from build123d import *

# Parameters (mm, degrees)
SKETCH1_W           = 94.925
SKETCH1_H           = 94.024999972
BOSS_EXTRUDE1_DEPTH = 127
BOSS_EXTRUDE2_DEPTH = 94.925
FILLET1_R           = 50.8
SHELL1_T            = -3
SKETCH3_W           = 94.925
SKETCH3_H           = 5
BOSS_EXTRUDE3_DEPTH = 16.999999878
SKETCH4_W           = 94.925
SKETCH4_H           = 5
BOSS_EXTRUDE4_DEPTH = 16.999999878
CUT_EXTRUDE1_REACH  = 365.178
SKETCH5_R           = 2.75


with BuildPart() as part:
    # Sketch1 → Boss-Extrude1 (new body)
    with BuildSketch(Plane.XY):
        Rectangle(SKETCH1_W, SKETCH1_H)
    extrude(amount=BOSS_EXTRUDE1_DEPTH)

    # Sketch2 → Boss-Extrude2 (add)
    with BuildSketch(Plane(origin=(47.4625, 0, 0), x_dir=(0, 0, -1), z_dir=(1, 0, 0))):
        Polygon((0, -47.012499986), (177.8, -199.412499986), (177.8, -105.387500014), (0, 47.012499986), align=None)
    extrude(amount=-BOSS_EXTRUDE2_DEPTH)

    # Fillet1
    fillet1_edges = [part.edges().sort_by_distance(p)[0] for p in [
        (0, -47.012499986, 0),
        (0, 47.012499986, 0),
    ]]
    fillet(fillet1_edges, radius=FILLET1_R)

    # Shell1
    shell1_openings = [part.faces().sort_by_distance(p)[0] for p in [
        (0, 0, 127),
        (0, -152.4, -177.8),
    ]]
    offset(amount=SHELL1_T, openings=shell1_openings, kind=Kind.INTERSECTION)

    # Sketch3 → Boss-Extrude3 (add)
    with BuildSketch(Plane(origin=(0, -47.012499986, 0), x_dir=(-1, 0, 0), z_dir=(0, -1, 0))):
        with Locations((0, -124.5)):
            Rectangle(SKETCH3_W, SKETCH3_H)
    extrude(amount=BOSS_EXTRUDE3_DEPTH)

    # Sketch4 → Boss-Extrude4 (add)
    with BuildSketch(Plane(origin=(0, 47.012499986, 0), x_dir=(1, 0, 0), z_dir=(0, 1, 0))):
        with Locations((0, -124.5)):
            Rectangle(SKETCH4_W, SKETCH4_H)
    extrude(amount=BOSS_EXTRUDE4_DEPTH)

    # Sketch5 → Cut-Extrude1 (cut, up to next)
    with BuildSketch(Plane(origin=(0, 0, 122), x_dir=(-1, 0, 0), z_dir=(0, 0, -1)), mode=Mode.PRIVATE) as cut_extrude1_sk1:
        with Locations((37.4625, 54.012499864)):
            Circle(SKETCH5_R)
    cut_extrude1_tool1 = extrude(cut_extrude1_sk1.sketch, amount=-CUT_EXTRUDE1_REACH, mode=Mode.PRIVATE) & part.part
    # Sketch5 → Cut-Extrude1 (cut, up to next)
    with BuildSketch(Plane(origin=(0, 0, 122), x_dir=(-1, 0, 0), z_dir=(0, 0, -1)), mode=Mode.PRIVATE) as cut_extrude1_sk2:
        with Locations((-37.4625, 54.012499864)):
            Circle(SKETCH5_R)
    cut_extrude1_tool2 = extrude(cut_extrude1_sk2.sketch, amount=-CUT_EXTRUDE1_REACH, mode=Mode.PRIVATE) & part.part
    # Sketch5 → Cut-Extrude1 (cut, up to next)
    with BuildSketch(Plane(origin=(0, 0, 122), x_dir=(-1, 0, 0), z_dir=(0, 0, -1)), mode=Mode.PRIVATE) as cut_extrude1_sk3:
        with Locations((37.4625, -54.012499864)):
            Circle(SKETCH5_R)
    cut_extrude1_tool3 = extrude(cut_extrude1_sk3.sketch, amount=-CUT_EXTRUDE1_REACH, mode=Mode.PRIVATE) & part.part
    # Sketch5 → Cut-Extrude1 (cut, up to next)
    with BuildSketch(Plane(origin=(0, 0, 122), x_dir=(-1, 0, 0), z_dir=(0, 0, -1)), mode=Mode.PRIVATE) as cut_extrude1_sk4:
        with Locations((-37.4625, -54.012499864)):
            Circle(SKETCH5_R)
    cut_extrude1_tool4 = extrude(cut_extrude1_sk4.sketch, amount=-CUT_EXTRUDE1_REACH, mode=Mode.PRIVATE) & part.part
    add(cut_extrude1_tool1.solids().sort_by_distance((-37.4625, 54.0125, 122))[0], mode=Mode.SUBTRACT)
    add(cut_extrude1_tool2.solids().sort_by_distance((37.4625, 54.0125, 122))[0], mode=Mode.SUBTRACT)
    add(cut_extrude1_tool3.solids().sort_by_distance((-37.4625, -54.0125, 122))[0], mode=Mode.SUBTRACT)
    add(cut_extrude1_tool4.solids().sort_by_distance((37.4625, -54.0125, 122))[0], mode=Mode.SUBTRACT)


solid = part.part
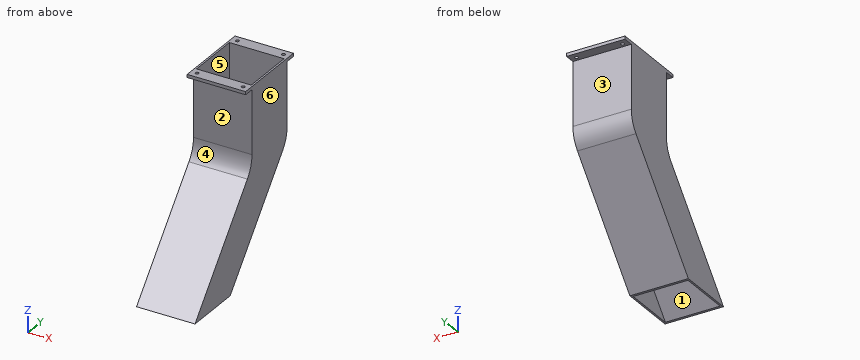
Here's how the part is built. I have some questions about the finished solid (model axes, mm). Face numbers are marked on the shaded views. A direction names the side the tool comes from. Give positions to 0.01 mm unless a question says otherwise; leave off trailing zeros. Order: outer loops, then holes, each group sorted by start corner. A loop starts at its lowest first (then second) coordinate and runs counter-clockwise, first axis right, second up. Notation, with made-up numbers: (-8, 86.5) -> (23, 86.5) arc R29 ccw to (23, 121.5) -> close; hole circle Ø4 at (56, 17). An arc over 180 degrees is marked (long way). Use a Markdown table: item, result. Add a question column.
Item 1: If we mould it in two halves opening along X, with no side actions, what happens to the marked faces 4, 5 and 6? For each: pulls with the +X half, pulls with the -X half, needs draft (parallel to the pull), parting line crosses it, or undercut.
Item 2: Imagine slicing it at B-B on z = 105. Please give me the cut outline in (x, y).
Item 3: Imagine slicing it at D-D on y = 19. Please give me the cut outline in (x, z).
Item 4: For the marked faces 1, 2 and 3, which set-ups out of +Z, -Z, +X, -X, +Y, -Y let a thin tool reach every point of the face, with its end or its side?
Item 5: Imagine slicing it at C-C on y = -94. Please give me the cut outline in (x, z).
Item 6: Will these pins go through, and if not, where does the flat tip stop? pin 1 (4 mm diameter, centred on x = 27.5, y = -39, fed in from -Z); pin 2 (6 mm diameter, centred on x = 19.5, y = -12, fed in from -Z); pin 3 (6.5 mm diameter, centred on x = 37.46, y = -54.01, fed in from +Z); pin 4 (18.5 mm diameter, centred on x = -20, y = -58, fed in from -Z).
Item 7: Imagine slicing it at A-A on x = 5. Please give me the cut outline in (y, z).
Item 8: I need wall thicknesses on line 1 (Y direction, x = 10, z = 45); line 2 (X direction, y = 35, z = 43.5); line 3 (Z direction, x = 33, y = -92.5). Which ranges of each line are inside material? Lowest first, please.
Data:
| question | item | result |
|---|---|---|
| 1 | face 4 | needs draft |
| 1 | face 5 | undercut |
| 1 | face 6 | pulls with the +X half |
| 2 | outline | (-47.46, -47.01) -> (47.46, -47.01) -> (47.46, 47.01) -> (-47.46, 47.01) -> close; hole (-44.46, -44.01) -> (44.46, -44.01) -> (44.46, 44.01) -> (-44.46, 44.01) -> close |
| 3 | outline | (-47.46, -32.68) -> (47.46, -32.68) -> (47.46, 127) -> (44.46, 127) -> (44.46, -28.07) -> (-44.46, -28.07) -> (-44.46, 127) -> (-47.46, 127) -> close |
| 4 | face 1 | none |
| 4 | face 2 | +X, -X, -Y |
| 4 | face 3 | -Z, +X, -X, +Y |
| 5 | outline | (-47.46, -164.51) -> (47.46, -164.51) -> (47.46, -54.82) -> (-47.46, -54.82) -> close; hole (-44.46, -159.9) -> (44.46, -159.9) -> (44.46, -59.43) -> (-44.46, -59.43) -> close |
| 6 | pin 1 | stops at z = -102.68 |
| 6 | pin 2 | stops at z = -72.35 |
| 6 | pin 3 | stops at z = 127 |
| 6 | pin 4 | stops at z = -133.31 |
| 7 | outline | (-199.41, -177.8) -> (-195.46, -177.8) -> (-56.96, -16.22) arc R53.8 ccw to (-44.01, 18.79) -> (-44.01, 127) -> (-64.01, 127) -> (-64.01, 122) -> (-47.01, 122) -> (-47.01, 18.79) arc R50.8 cw to (-59.24, -14.27) -> close; (-109.34, -177.8) -> (-105.39, -177.8) -> (34.78, -14.27) arc R50.8 ccw to (47.01, 18.79) -> (47.01, 122) -> (64.01, 122) -> (64.01, 127) -> (44.01, 127) -> (44.01, 18.79) arc R47.8 cw to (32.5, -12.32) -> close |
| 8 | line 1 | y = -47.01 to -44.01, 44.01 to 47.01 |
| 8 | line 2 | x = -47.46 to -44.46, 44.46 to 47.46 |
| 8 | line 3 | z = -162.76 to -158.15, -57.68 to -53.07 |
